For this review, use the dimensioned drawing (mm, ordinates from the lowest corner) and the shaded views. A direction names the side the tool comes from. Give positions to 0.01 mm unless a question says otherwise; leave off trailing zeros. Loops run counter-clockwise (first coordinate to the right, second up) from the corner with the lowest first, then second, coordinate; pieces in that order, holes last. Notation, with made-up numbers: (-23, 77.5) -> (11, 77.5) arc R24 ccw to (11, 87.5) -> close; hole circle Ø8 at (-33, -15). An arc over 180 degrees is marked (long way). Use a Markdown table: item, result. Add a question column.
1. For pin 1 Ø8 at (y, z) = (34.5, 69) entering from -X; pin 2 Ø4 at (y, z) = (11.5, 18) entering from -X; pin 3 Ø12 at (x, y) = (33.5, 6) entering from -Z; pin 4 Ø4 at (x, y) = (23, 19.5) entering from -Z, all flat-tipped, find the tip position at first contact; note any pin that passes through.
2. Add section A-A (x = 25). State the section outline as (y, z) points, and give its area (3 significant figures).
3. Add section B-B (y = 25.5). State the section outline as (x, z) points, and give its area (4 significant figures).
4. For the marked faces 1 and 2, list the 3-axis set-ups (+Z, -Z, +X, -X, +Y, -Y) from which the entire face can be reached by the end or side of a thin tool; tool diameter is ignored.
5. To check wall thickness, follow line 1 (Y direction, x = 15, z = 53); line 2 (Z direction, x = 24, y = 33); line 3 (Z direction, x = 30.5, y = 10.5). State the ranges of each line that lie inside material, in increasing order.
6. Add section C-C (z = 50). State the section outline as (x, y) points (1 decimal).
7. Add section D-D (y = 12). State the section outline as (x, z) points.
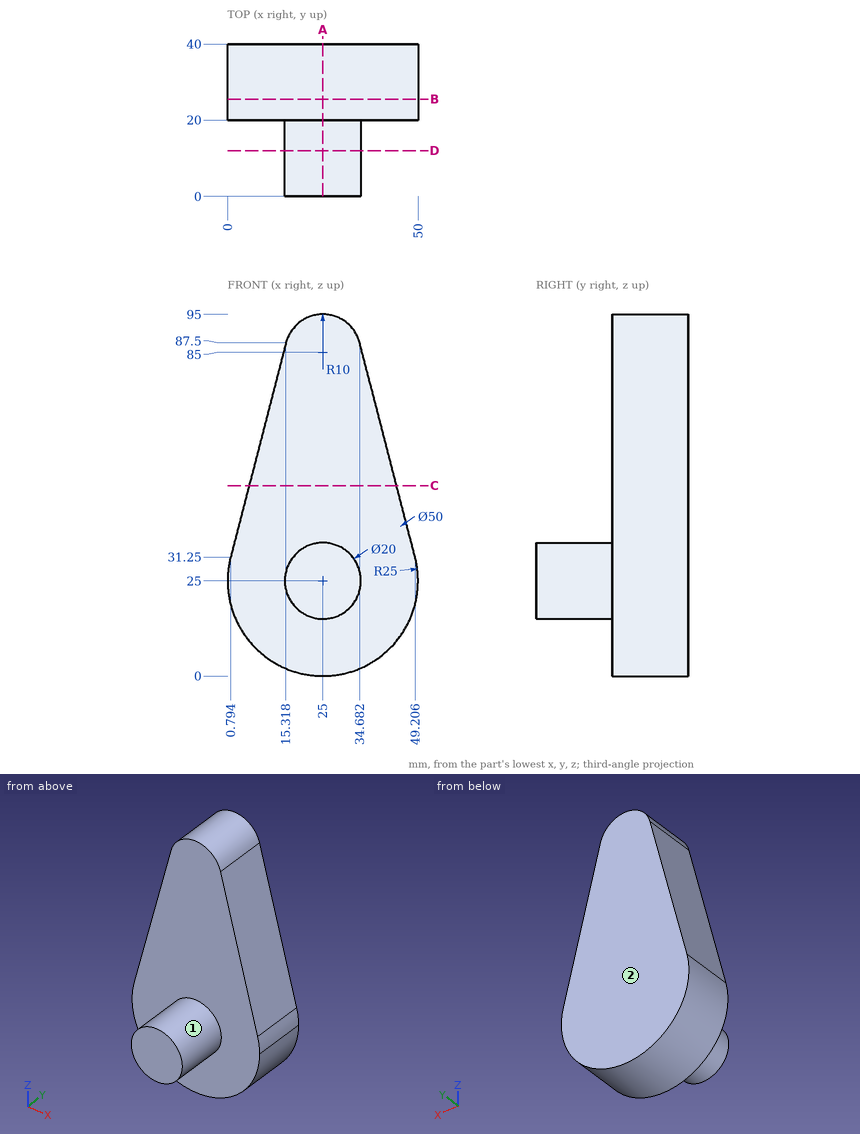
Taken from the geometry:
| question | item | result |
|---|---|---|
| 1 | pin 1 | stops at x = 9.51 |
| 1 | pin 2 | stops at x = 16.34 |
| 1 | pin 3 | stops at z = 15.32 |
| 1 | pin 4 | stops at z = 0 |
| 2 | outline | (0, 15) -> (20, 15) -> (20, 0) -> (40, 0) -> (40, 95) -> (20, 95) -> (20, 35) -> (0, 35) -> close |
| 2 | area | 2,300 mm^2 |
| 3 | outline | (0.79, 31.25) arc R25 ccw (long way) to (50, 25) arc R25 ccw to (49.21, 31.25) -> (34.68, 87.5) arc R10 ccw to (15.32, 87.5) -> close |
| 3 | area | 3,305 mm^2 |
| 4 | face 1 | -Y |
| 4 | face 2 | +Z, -Z, +X, -X, +Y |
| 5 | line 1 | y = 20 to 40 |
| 5 | line 2 | z = 0.02 to 94.95 |
| 5 | line 3 | z = 16.65 to 33.35 |
| 6 | outline | (5.6, 20) -> (44.4, 20) -> (44.4, 40) -> (5.6, 40) -> close |
| 7 | outline | circle Ø20 at (25, 25) |
